For this review, take the finished solid that the model builds, in its own axes (mm). A direction names the side the tool comes from. Give positions to 0.01 mm unless a question says otherwise; leave off trailing zeros. Write each loop counter-clockwise with the first axis right and the second up, starting at its lowest first coordinate (ties: lowest second). Pieces come first, ordered by that corner, then holes. Notation, with made-up numbers: M -31,24 L -21,24 A12 ccw -21,44 Z; hole C 11.25,63 d9. An arc over 180 degrees is marked long. Use one line per item in the form item = value. Start each with the question number.
Q1. Tool access review of faces 4 (the flat face through (7.5, -49, 45)), 5 (the flat face through (22.5, -40, 37)), 6 (the flat face through (-43, 17, 37)): name each direction out of +Z, -Z, +X, -X, +Y, -Y from which nothing blocks a thin tool from reaching the whole face with its end or side.
Q2. Mouldability with a two-part tool opening along Y and no side actions: class faces 1 (the cylindrical face through (-47.846, 2.253, 36.975)), 2 (the cylindrical face through (-72, 0, 37)), 3 (the flat face through (-19, -9, 0)) as released by +Y, released by -Y, zero draft, split by the parting line, or undercut.
Q3. Consider section C-C on x = -61. Write out the cut boundary in (y, z).
Q4. For probe 1 along X at (y, z) = (6, 48); probe 2 along X at (y, z) = (1.5, 5); probe 3 along Y at (x, z) = (-55, 56), list the stretches that pass through material, from the lowest coordinate up. Write a range as [from, to].
Q5. Consider section B-B on z = 39.5. Write out the cut boundary in (x, y) (3 decimals).
Q6. Clearance check with flat-ended pins moving along their axes: pin 1 Ø5 at (y, z) = (7, 44) entering from -X; pin 2 Ø24 at (x, y) = (0, 0) entering from -Z; pin 3 Ø3 at (x, z) = (-28, 48.5) entering from +Y; pin 4 Ø23 at (y, z) = (-52.25, 36.36) entering from +X. State where each tip first meets the part, or that it passes through.
Q7. Consider section D-D on y = -40.5. Write out the cut boundary in (x, z).
Q8. Consider section A-A on y = 0. Write out the cut boundary in (x, z).
```python
from build123d import *

# Parameters (mm, degrees)
SKETCH1_R           = 7.5
SKETCH1_R_2         = 20
BOSS_EXTRUDE1_DEPTH = 75
BOSS_EXTRUDE2_DEPTH = 75
FILLET6_R           = 34
FILLET8_R           = 34
SKETCH3_R           = 8.750256672
CUT_EXTRUDE1_DEPTH  = 15


with BuildPart() as part:
    # Sketch1 → Boss-Extrude1 (new body)
    with BuildSketch(Plane.XY):
        with BuildLine():
            Line((-30.594117082, 17), (-55, 17))
            ThreePointArc((-55, 17), (-72, 0), (-55, -17))
            Line((-55, -17), (-30.594117082, -17))
            ThreePointArc((-30.594117082, -17), (35, 0), (-30.594117082, 17))
        make_face()
        with Locations((-55, 0)):
            Circle(SKETCH1_R, mode=Mode.SUBTRACT)
        Circle(SKETCH1_R_2, mode=Mode.SUBTRACT)
    extrude(amount=BOSS_EXTRUDE1_DEPTH)

    # Sketch1_12 → Boss-Extrude2 (add)
    with BuildSketch(Plane.XY):
        with BuildLine():
            Line((22.5, -72), (22.5, -26.809513237))
            ThreePointArc((22.5, -26.809513237), (15.446901808, -31.406897722), (7.5, -34.186985828))
            Line((7.5, -34.186985828), (7.5, -72))
            Line((7.5, -72), (22.5, -72))
        make_face()
        with BuildLine():
            ThreePointArc((-7.5, -34.186985828), (-15.446901808, -31.406897722), (-22.5, -26.809513237))
            Line((-22.5, -26.809513237), (-22.5, -72))
            Line((-22.5, -72), (-7.5, -72))
            Line((-7.5, -72), (-7.5, -34.186985828))
        make_face()
    extrude(amount=BOSS_EXTRUDE2_DEPTH)

    # Fillet6
    fillet6_edges = [part.edges().sort_by_distance(p)[0] for p in [
        (-15, -72, 0),
        (-15, -72, 75),
    ]]
    fillet(fillet6_edges, radius=FILLET6_R)

    # Fillet8
    fillet8_edges = [part.edges().sort_by_distance(p)[0] for p in [
        (15, -72, 75),
        (15, -72, 0),
    ]]
    fillet(fillet8_edges, radius=FILLET8_R)

    # Sketch3 → Cut-Extrude1 (cut)
    with BuildSketch(Plane(origin=(22.5, 0, 0), x_dir=(0, 0, -1), z_dir=(1, 0, 0))):
        with Locations(Location((-36.363077214, -52.246350357, 0), (0, 0, 90))):
            Circle(SKETCH3_R)
    cut_extrude1 = extrude(amount=-CUT_EXTRUDE1_DEPTH, mode=Mode.SUBTRACT)

    # Mirror2: Cut-Extrude1 across plane
    add(cut_extrude1.mirror(Plane(origin=(0, 0, 0), x_dir=(0, 0, 1), z_dir=(1, 0, 0))), mode=Mode.SUBTRACT)


solid = part.part
```
Working result:
q1.face_4 = +Z, -Z, -Y
q1.face_5 = +Z, -Z, +X, -Y
q1.face_6 = +Z, -Z, -X, +Y
q2.face_1 = undercut
q2.face_2 = split by the parting line
q2.face_3 = zero draft
q3.outline = M -15.91,0 L -4.5,0 L -4.5,75 L -15.91,75 Z; M 4.5,0 L 15.91,0 L 15.91,75 L 4.5,75 Z
q4.probe_1 = [-70.91, -59.5], [-50.5, -19.08], [19.08, 34.48]
q4.probe_2 = [-71.93, -62.35], [-47.65, -19.94], [19.94, 34.97]
q4.probe_3 = [-17, -7.5], [7.5, 17]
q5.outline = M -55,-17 L -30.594,-17 A35 ccw -22.5,-26.81 L -22.5,-44.078 L -7.5,-44.078 L -7.5,-34.187 A35 ccw 7.5,-34.187 L 7.5,-44.078 L 22.5,-44.078 L 22.5,-26.81 A35 ccw long -30.594,17 L -55,17 A17 ccw Z; M -22.5,-72 L -7.5,-72 L -7.5,-60.415 L -22.5,-60.415 Z; M 7.5,-72 L 22.5,-72 L 22.5,-60.415 L 7.5,-60.415 Z; hole C -55,0 d15; hole C 0,0 d40
q6.pin_1 = -71.39
q6.pin_2 = through
q6.pin_3 = 22.86
q6.pin_4 = 22.5
q7.outline = M -22.5,0.09 L -7.5,0.09 L -7.5,74.91 L -22.5,74.91 Z; M 7.5,0.09 L 22.5,0.09 L 22.5,74.91 L 7.5,74.91 Z
q8.outline = M -72,0 L -62.5,0 L -62.5,75 L -72,75 Z; M -47.5,0 L -20,0 L -20,75 L -47.5,75 Z; M 20,0 L 35,0 L 35,75 L 20,75 Z
